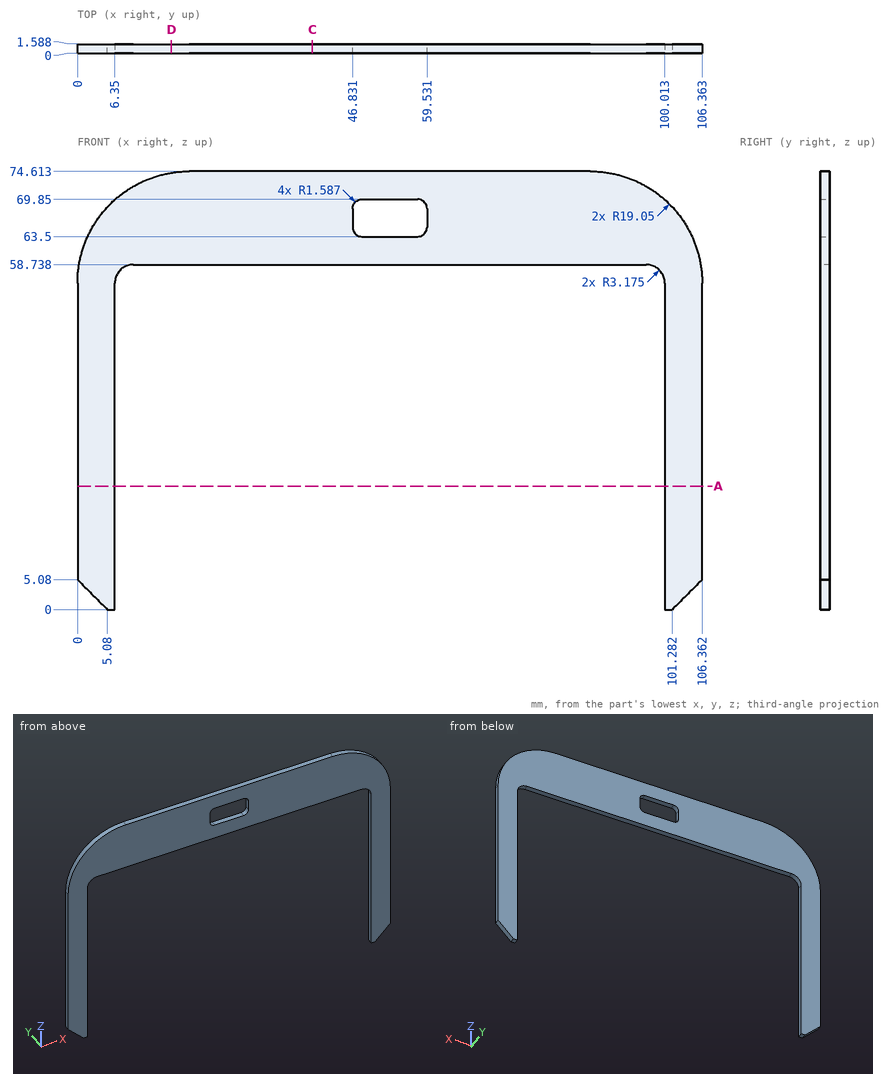
Verification items for this drawing (mm, ordinates from the low corner). Coordinates: 2 decimals unless noted, no trailing zeros. Write each loop counter-clockwise with the first axis right and the second up, starting at its lowest first coordinate (ties: lowest second). Pieces come first, ordered by that corner, then holes. Notation, with made-up numbers: (53.5, 80.25) -> (107.5, 80.25) arc R23 cw to (107.5, 100.25) -> close; hole circle Ø2 at (50.5, 66). An arc over 180 degrees is marked (long way). One line per item, written item: value. Start each with the question number.
Q1. Go/stop test with a flat-tipped pin: P1, Ø0.5, axis at x = 71, y = 1, coming from the -Z side. Record where the tip stops, or that it passes through.
Q2. Thickness scan on L1, parallel to X at y = 0.6, z = 5.5; L2, parallel to Z at x = 56.5, y = 1.2; L3, parallel to Z at x = 21.5, y = 1.2. Record the ranges inside material, lowest first. Write a range as from..to.
Q3. Cross-section at A-A on z = 21. Enter the section's corners in (x, y).
Q4. Cross-section at D-D on x = 16. Enter the section's corners in (y, z).
Q5. Cross-section at C-C on x = 40. Enter the section's corners in (y, z).
Checked values:
1. P1: stops at z = 58.74
2. L1: x = 0..6.35, 100.01..106.36
2. L2: z = 58.74..63.5, 69.85..74.61
2. L3: z = 58.74..74.61
3. outline: (0, 0) -> (6.35, 0) -> (6.35, 1.59) -> (0, 1.59) -> close; (100.01, 0) -> (106.36, 0) -> (106.36, 1.59) -> (100.01, 1.59) -> close
4. outline: (0, 58.74) -> (1.59, 58.74) -> (1.59, 74.37) -> (0, 74.37) -> close
5. outline: (0, 58.74) -> (1.59, 58.74) -> (1.59, 74.61) -> (0, 74.61) -> close
